Geometry check sheet. Reference: the model listing, model coordinates, mm. A direction names the side the tool comes from. Give positions to 0.01 mm unless a question says otherwise; leave off trailing zeros. Order: outer loops, then holes, each group sorted by start corner. A loop starts at its lowest first (then second) coordinate and runs counter-clockwise, first axis right, second up. Notation, with made-up numbers: M 55,60 L 70,60 A9 cw 70,75 Z; hole C -20,81 d9. An arc over 180 degrees is marked long. One line per question, with ' | ' between items. Start each with the question number.
from build123d import *

# Parameters (mm, degrees)
SKETCH1_W               = 254
SKETCH1_H               = 304.8
BOSS_EXTRUDE1_DEPTH     = 10
CUT_EXTRUDE1_DEPTH      = 2.5
SKETCH3_W               = 15
SKETCH3_H               = 100
BOSS_EXTRUDE2_DEPTH     = 20
CUT_EXTRUDE4_DEPTH      = 262.907148317
CUT_EXTRUDE4_DEPTH_BACK = 262.907148317
SKETCH4_W               = 7.192307822
SKETCH4_H               = 86.692915772
FILLET2_R               = 10


with BuildPart() as part:
    # Sketch1 → Boss-Extrude1 (new body)
    with BuildSketch(Plane.XY):
        Rectangle(SKETCH1_W, SKETCH1_H)
    extrude(amount=BOSS_EXTRUDE1_DEPTH)

    # Sketch2 → Cut-Extrude1 (cut)
    with BuildSketch(Plane.XY.offset(10)):
        with BuildLine():
            Line((-62, -137.4), (62, -137.4))
            ThreePointArc((62, -137.4), (97.355339059, -122.755339059), (112, -87.4))
            Line((112, -87.4), (112, 87.4))
            ThreePointArc((112, 87.4), (97.355339059, 122.755339059), (62, 137.4))
            Line((62, 137.4), (-62, 137.4))
            ThreePointArc((-62, 137.4), (-97.355339059, 122.755339059), (-112, 87.4))
            Line((-112, 87.4), (-112, -87.4))
            ThreePointArc((-112, -87.4), (-97.355339059, -122.755339059), (-62, -137.4))
        make_face()
    extrude(amount=-CUT_EXTRUDE1_DEPTH, mode=Mode.SUBTRACT)

    # Sketch3 → Boss-Extrude2 (add)
    with BuildSketch(Plane.XY.offset(7.5)):
        with Locations((76.718712096, 0)):
            Rectangle(SKETCH3_W, SKETCH3_H)
    extrude(amount=BOSS_EXTRUDE2_DEPTH)

    # Sketch4 → Cut-Extrude4 (cut, two sides: drawn at the far end of the back side and taken through both)
    with BuildSketch(Plane(origin=(84.218712096, 0, 0), x_dir=(0, 0, -1), z_dir=(1, 0, 0)).offset(-CUT_EXTRUDE4_DEPTH_BACK)):
        with Locations((-18.014845045, 0)):
            Rectangle(SKETCH4_W, SKETCH4_H)
    extrude(amount=CUT_EXTRUDE4_DEPTH + CUT_EXTRUDE4_DEPTH_BACK, mode=Mode.SUBTRACT)

    # Fillet2
    fillet2_edges = [part.edges().sort_by_distance(p)[0] for p in [
        (76.718712096, 50, 27.5),
        (76.718712096, -50, 27.5),
    ]]
    fillet(fillet2_edges, radius=FILLET2_R)


solid = part.part
Item 1: Depth check by flat-ended pin: pin 1 (3 mm diameter, centred on x = 74.5, y = -92, fed in from +Z); pin 2 (3.5 mm diameter, centred on x = 76, z = 18, fed in from +Y); pin 3 (3 mm diameter, centred on x = 74.5, z = 13, fed in from -Y). Enter the tip coordinate at first touch or a pass-through.
Item 2: Material ranges on line 1 along X through (y, z) = (25, 9.5); line 2 along Z through (x, y) = (-60.5, 89); line 3 along X through (y, z) = (12.5, 25.5), recorded low to high.
Item 3: Cross-section at A-A, the plane y = 2. Record the cut outline in (x, z), plus the area to 3 significant figures.
Item 4: Cross-section at B-B, the plane x = 23. Record the cut outline in (y, z), plus the area to 3 significant figures.
Item 5: Set-up check for faces 1 (the cylindrical face through (96.964, -123.142, 8.768)), 2 (the flat face through (77, -1, 21.611)), 3 (the flat face through (77, 1, 27.5)): record each of +Z, -Z, +X, -X, +Y, -Y from which the full face is reachable in a straight line by a thin tool's end or side.
Item 6: Cross-section at C-C, the plane y = -62.5. Record the cut outline in (x, z).
Item 7: Mould release check, pull along Y, two halves, no side actions. Record for faces 4 (the flat face through (-2, -152.4, 5)), 5 (the flat face through (-2, 152.4, 5)), 6 (the flat face through (127, -2, 5)), 7 (the cylindrical face through (-96.964, 123.142, 8.768)): released by +Y, released by -Y, zero draft, split by the parting line, or undercut.
Outcome:
1) pin 1: stops at z = 7.5 | pin 2: stops at y = 50 | pin 3: stops at y = -50
2) line 1: x = -127 to -112, 69.22 to 84.22, 112 to 127 | line 2: z = 0 to 7.5 | line 3: x = 69.22 to 84.22
3) outline: M -127,0 L 127,0 L 127,10 L 112,10 L 112,7.5 L 84.22,7.5 L 84.22,14.42 L 69.22,14.42 L 69.22,7.5 L -112,7.5 L -112,10 L -127,10 Z; M 69.22,21.61 L 84.22,21.61 L 84.22,27.5 L 69.22,27.5 Z | area: 2,170 mm²
4) outline: M -152.4,0 L 152.4,0 L 152.4,10 L 137.4,10 L 137.4,7.5 L -137.4,7.5 L -137.4,10 L -152.4,10 Z | area: 2,360 mm²
5) face 1: +Z | face 2: +X, -X | face 3: +Z, +X, -X, +Y, -Y
6) outline: M -127,0 L 127,0 L 127,10 L 112,10 L 112,7.5 L -112,7.5 L -112,10 L -127,10 Z
7) face 4: released by -Y | face 5: released by +Y | face 6: zero draft | face 7: undercut
